Job drawing, mm, ordinate dimensions from the low corner. One solid piece. Give positions to 0.01 mm unless a question says otherwise; leave off trailing zeros. Order: outer loops, then holes, each group sorted by start corner. A loop starts at its lowest first (then second) coordinate and runs counter-clockwise, first axis right, second up.
1. Slice it at C-C on x = 50. List the corners of the cut face in (y, z).
2. Probe line 1 (Y direction, x = 11.5, z = 2.1); line 2 (X direction, y = 40.5, z = 2.3) (1 decimal); line 3 (X direction, y = 7, z = 0.4) (1 decimal). List the from-to ranges inside material, lowest first.
3. Slice it at A-A on x = 17.5. List the corners of the cut face in (y, z).
4. Drop a flat-ended pin along its axis: pin 1 Ø1.8 at (x, y) = (11.5, 14) entering from +Z. Give the stop position or say it passes through.
5. Slice it at B-B on z = 2.15. Give the number of separate pieces and of enclosed holes in the cut face, and give its area (3 significant figures).
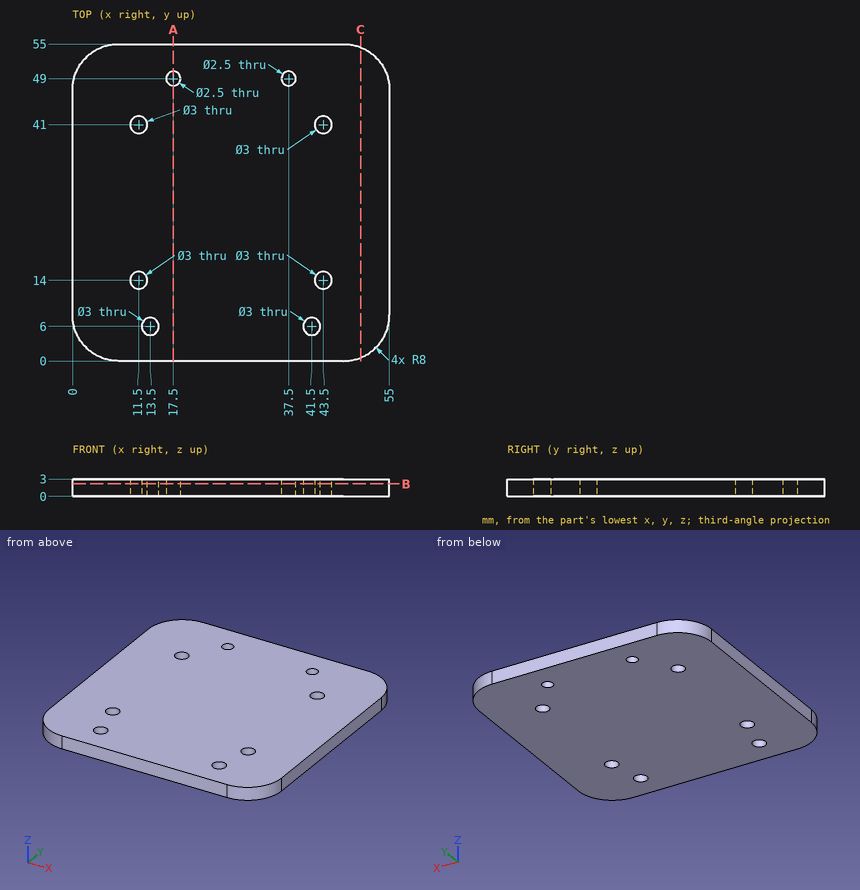
Data:
1. outline: (0.58, 0) - (54.42, 0) - (54.42, 3) - (0.58, 3) - close
2. line 1: y = 0 to 12.5, 15.5 to 39.5, 42.5 to 55
2. line 2: x = 0 to 10.1, 12.9 to 42.1, 44.9 to 55
2. line 3: x = 0.1 to 12.4, 14.6 to 40.4, 42.6 to 54.9
3. outline: (0, 0) - (47.75, 0) - (47.75, 3) - (0, 3) - close; (50.25, 0) - (55, 0) - (55, 3) - (50.25, 3) - close
4. pin 1: passes through
5. separate pieces: 1
5. enclosed holes: 8
5. area: 2,920 mm2
